```python
from build123d import *

# Parameters (mm, degrees)
P_IDAT_VYSUNUT_M1_DEPTH = 1
ZAOBLIT1_R              = 1


with BuildPart() as part:
    # Skica1 → Přidat vysunutím1 (new body)
    with BuildSketch(Plane.XY):
        with BuildLine():
            Line((-0.5, -3.211308145), (-0.5, -6.982120022))
            ThreePointArc((-0.5, -6.982120022), (0, 7), (0.5, -6.982120022))
            Line((0.5, -6.982120022), (0.5, -3.211308145))
            ThreePointArc((0.5, -3.211308145), (0, 3.25), (-0.5, -3.211308145))
        make_face()
    extrude(amount=P_IDAT_VYSUNUT_M1_DEPTH)

    # Zaoblit1
    zaoblit1_edges = [part.edges().sort_by_distance(p)[0] for p in [
        (-0.5, -3.211308145, 0.5),
        (-0.5, -6.982120022, 0.5),
        (0.5, -6.982120022, 0.5),
        (0.5, -3.211308145, 0.5),
    ]]
    fillet(zaoblit1_edges, radius=ZAOBLIT1_R)


solid = part.part
```
Verification items for the finished model (mm, model axes). A direction names the side the tool comes from. Round coordinates to 2 decimals unless told otherwise and drop trailing zeros. Write each loop counter-clockwise with the first axis right and the second up, starting at its lowest first coordinate (ties: lowest second). Pieces come first, ordered by that corner, then holes. Notation, with made-up numbers: (5.5, 37) - (52.5, 37) arc R14 cw to (52.5, 43) - close; hole circle Ø8 at (5.5, 87). An arc over 180 degrees is marked (long way). Answer as a JSON object with one key per item and string values. Group by question number.
Q1. Mould release check, pull along X, two halves, no side actions. Record for faces 4 (the flat face through (-1.5, 3.3, 0)), 5 (the flat face through (0.5, -4.9, 0.5)), 6 (the cylindrical face through (-0.283, 6.994, 0.493)): released by +X, released by -X, zero draft, split by the parting line, or undercut.
Q2. Thickness scan on line 1 (X direction, y = 0, z = 0.8); line 2 (Y direction, x = 0, z = 0.55); line 3 (Y direction, x = 1, z = 0.6). Record the ranges inside material, lowest first.
Q3. Section check D-D, the plane x = 0. Enter the section's corners in (y, z).
Q4. Tool access check on faces 1 (the cylindrical face through (0.673, -3.415, 0.507)), 2 (the flat face through (-1.5, 3.3, 1)), 3 (the flat face through (-0.5, -4.9, 0.5)). Record the directions out of +Z, -Z, +X, -X, +Y, -Y that give a thin tool (end or side, any length) a straight path to the whole face; none if there is none.
Q5. Section check A-A, the plane y = 0. Enter the section's corners in (x, z), plus the area to 3 significant figures.
Q6. Section check B-B, the plane z = 0.2. Enter the section's corners in (x, y), plus the area to 3 significant figures.
Q7. Section check C-C, the plane x = 3. Enter the section's corners in (y, z), plus the area to 3 significant figures.
Found:
{
 "1": {"face 4": "zero draft", "face 5": "undercut", "face 6": "split by the parting line"},
 "2": {"line 1": "x = -7 to -3.25, 3.25 to 7", "line 2": "y = 3.25 to 7", "line 3": "y = -6.68 to -3.11, 3.09 to 6.93"},
 "3": {"outline": "(3.25, 0) - (7, 0) - (7, 1) - (3.25, 1) - close"},
 "4": {"face 1": "+Z, -Z", "face 2": "+Z, +X, -X, +Y, -Y", "face 3": "+Z, -Z, -Y"},
 "5": {"outline": "(-7, 0) - (-3.25, 0) - (-3.25, 1) - (-7, 1) - close; (3.25, 0) - (7, 0) - (7, 1) - (3.25, 1) - close", "area": "7.50 mm^2"},
 "6": {"outline": "(-1.75, -6.78) arc R1 ccw to (-0.5, -5.81) - (-0.5, -3.98) arc R1 ccw to (-1.15, -3.04) arc R3.25 cw (long way) to (1.15, -3.04) arc R1 ccw to (0.5, -3.98) - (0.5, -5.81) arc R1 ccw to (1.75, -6.78) arc R7 ccw (long way) to start", "area": "116 mm^2"},
 "7": {"outline": "(-6.32, 0) - (-1.25, 0) - (-1.25, 1) - (-6.32, 1) - close; (1.25, 0) - (6.32, 0) - (6.32, 1) - (1.25, 1) - close", "area": "10.1 mm^2"}
}
